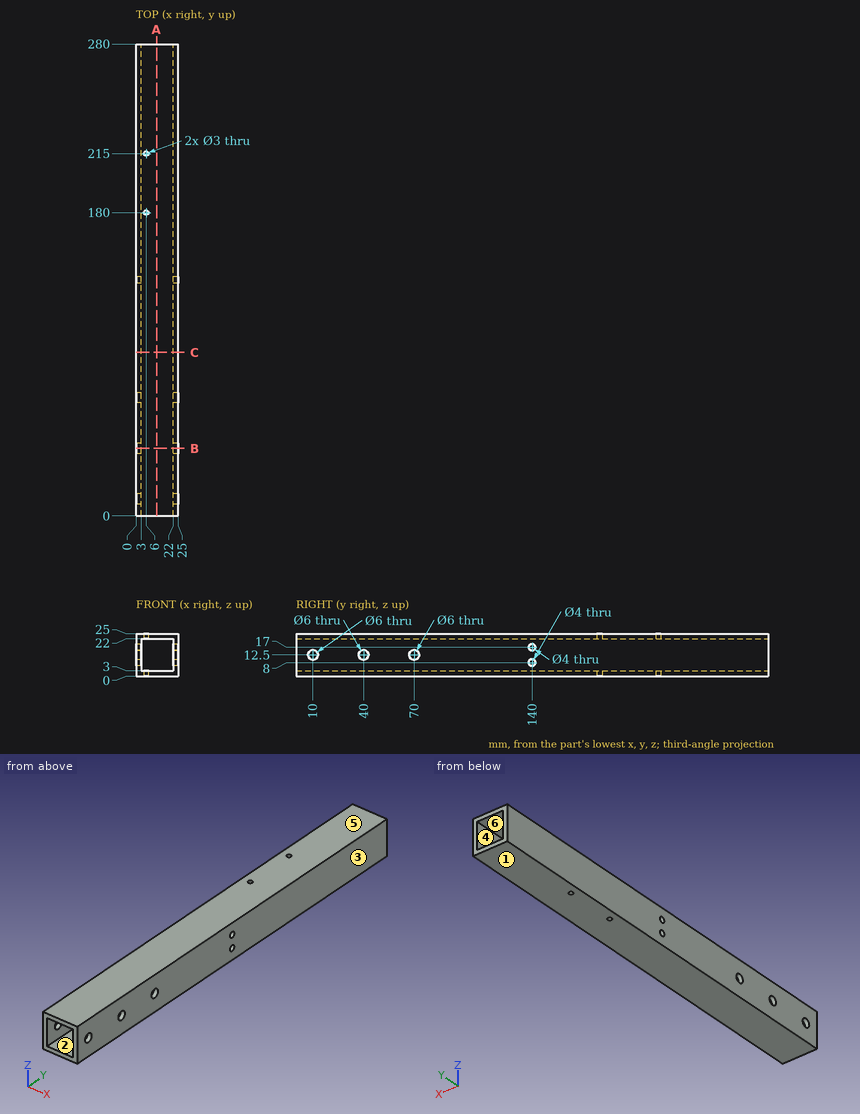
Check sheet for the drawn part. Datum: minimum x, y, z corner. Units: mm. A direction names the side the tool comes from. Give positions to 0.01 mm unless a question says otherwise; leave off trailing zeros. Order: outer loops, then holes, each group sorted by start corner. A loop starts at its lowest first (then second) coordinate and runs counter-clockwise, first axis right, second up. Notation, with made-up numbers: (33.25, 88.25) -> (91.25, 88.25) arc R4 cw to (91.25, 92.25) -> close; hole circle Ø4 at (64.25, 68.25). An arc over 180 degrees is marked (long way). Use a Markdown table: item, result.
1) Section check A-A, the plane x = 12.25. Record the boundary of the cut face in (y, z).
Results:
| item | result |
|---|---|
| outline | (0, 0) -> (280, 0) -> (280, 3) -> (0, 3) -> close; (0, 22) -> (280, 22) -> (280, 25) -> (0, 25) -> close |
2) Material ranges on probe 1 along Y at (x, z) = (6, 22.7); probe 2 along X at (y, z) = (180, 1.05); probe 3 along X at (y, z) = (58.5, 17.75), recorded low to high.
Results:
| item | result |
|---|---|
| probe 1 | 0 to 178.5, 181.5 to 213.5, 216.5 to 280 |
| probe 2 | 0 to 4.5, 7.5 to 25 |
| probe 3 | 0 to 3, 22 to 25 |
3) Section check C-C, the plane y = 97. Record the boundary of the cut face in (x, z), then the cut area to 3 significant figures.
Results:
| item | result |
|---|---|
| outline | (0, 0) -> (25, 0) -> (25, 25) -> (0, 25) -> close; hole (3, 3) -> (22, 3) -> (22, 22) -> (3, 22) -> close |
| area | 264 mm² |
4) Section check B-B, the plane y = 40. Record the boundary of the cut face in (x, z).
Results:
| item | result |
|---|---|
| outline | (0, 0) -> (25, 0) -> (25, 9.5) -> (22, 9.5) -> (22, 3) -> (3, 3) -> (3, 9.5) -> (0, 9.5) -> close; (0, 15.5) -> (3, 15.5) -> (3, 22) -> (22, 22) -> (22, 15.5) -> (25, 15.5) -> (25, 25) -> (0, 25) -> close |
5) Mould release check, pull along Z, two halves, no side actions. Record for the marked faces 1, 2, 3 and 4: pulls with the +Z half, pulls with the -Z half, needs draft (parallel to the pull), parting line crosses it, or undercut.
Results:
| item | result |
|---|---|
| face 1 | pulls with the -Z half |
| face 2 | undercut |
| face 3 | needs draft |
| face 4 | undercut |
6) Tool access check on the marked faces 5 and 6. Record the directions out of +Z, -Z, +X, -X, +Y, -Y that give a thin tool (end or side, any length) a straight path to the whole face; none if there is none.
Results:
| item | result |
|---|---|
| face 5 | +Z, +X, -X, +Y, -Y |
| face 6 | +Y, -Y |
